```python
from build123d import *

# Parameters (mm, degrees)
F1_DEPTH = 43


with BuildPart() as f1:
    # F0 (on Front) → F1 (new body)
    with BuildSketch(Plane.XZ):
        with BuildLine():
            ThreePointArc((-7, 0), (0, -7), (7, 0))
            ThreePointArc((7, 0), (0, 7), (-7, 0))
        make_face()
        with BuildLine():
            Line((-14, 11), (-14, 0))
            Line((-14, 0), (-14, -7))
            Line((-14, -7), (-7, -14))
            Line((-7, -14), (0, -14))
            Line((0, -14), (21.066626, -14))
            ThreePointArc((21.066626, -14), (24.331862, -15.213414), (26.012265, -18.264706))
            ThreePointArc((26.012265, -18.264706), (28.349095, -26.115672), (32.788067, -33))
            Line((32.788067, -33), (38, -33))
            Line((38, -33), (67, 0))
            Line((67, 0), (67, 19))
            Line((67, 19), (65.127473, 23.242816))
            Line((65.127473, 23.242816), (41.127473, 23.242816))
            ThreePointArc((41.127473, 23.242816), (32.713444, 15.660003), (21.479572, 14.212572))
            Line((21.479572, 14.212572), (0, 18))
            Line((0, 18), (-7, 18))
            Line((-7, 18), (-14, 11))
        make_face()
        with BuildLine():
            ThreePointArc((-7, 0), (0, 7), (7, 0))
            ThreePointArc((7, 0), (0, -7), (-7, 0))
        make_face(mode=Mode.SUBTRACT)
    extrude(amount=F1_DEPTH)


solid = f1.part
```
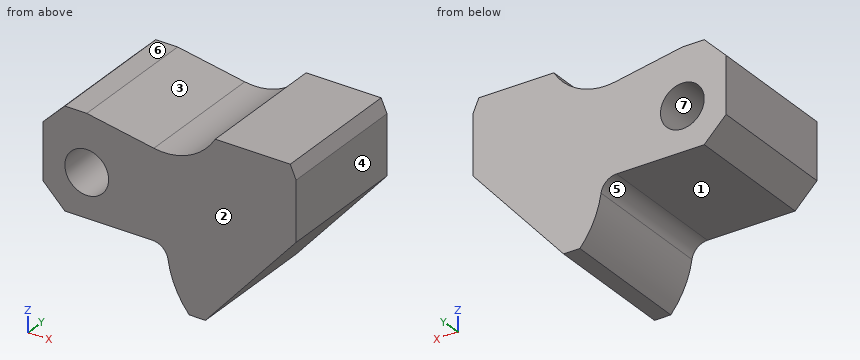
Here's how the part is built. I have some questions about the finished solid (model axes, mm). Face numbers are marked on the shaded views. A direction names the side the tool comes from. Give positions to 0.01 mm unless a question says otherwise; leave off trailing zeros. Order: outer loops, then holes, each group sorted by start corner. A loop starts at its lowest first (then second) coordinate and runs counter-clockwise, first axis right, second up. Notation, with made-up numbers: (35, 22) - (94, 22) arc R14 ccw to (94, 44) - close; hole circle Ø2 at (-8.5, -34.75). An arc over 180 degrees is marked (long way). Answer as a JSON object with one key per item and string values. Group by question number.
Item 1: If we mould it in two halves opening along Z, with no side actions, what happens to the marked faces 4, 5, 6 and 7? For each: pulls with the +Z half, pulls with the -Z half, needs draft (parallel to the pull), parting line crosses it, or undercut.
Item 2: Which directions (+Z, -Z, +X, -X, +Y, -Y) give clear straight access to the entire face, cutting with the end or side of a thin tool? Please do the marked faces 1, 2 and 3.
Item 3: If we section it at D-D on z = -27: Please give me the cut outline in (x, y).
Item 4: For P1, Ø5, axis at y = -20, z = -12.5, coming from the -X side; P2, Ø1, axis at y = -9.5, z = -25.5, coming from the -X side; P3, Ø2, axis at x = 1, y = -22.5, coming from the -Z side, each with a flat end and sliding along its axis, tell me the tip position at first contact or that it passes through.
Item 5: If we section it at B-B on z = -1: Please give me the cut outline in (x, y), and give its area (3 significant figures).
Item 6: If we section it at C-C on x = 13: Please give me the cut outline in (y, z).
Item 7: Please list where these lines run through material, in increasing order: probe 1 along Z at (x, y) = (0, -30); probe 2 along X at (y, z) = (-24, 0); probe 3 along X at (y, z) = (-32.5, 5).
Item 8: If we section it at A-A on y = -4: Please give me the cut outline in (x, z).
Result set:
{
 "1": {"face 4": "needs draft", "face 5": "pulls with the -Z half", "face 6": "pulls with the +Z half", "face 7": "undercut"},
 "2": {"face 1": "-Z, -X, +Y, -Y", "face 2": "+Z, -Z, +X, -X, -Y", "face 3": "+Z, +Y, -Y"},
 "3": {"outline": "(28.77, -43) - (43.27, -43) - (43.27, 0) - (28.77, 0) - close"},
 "4": {"P1": "x = -11", "P2": "x = 27.86", "P3": "z = -14"},
 "5": {"outline": "(-14, -43) - (-6.93, -43) - (-6.93, 0) - (-14, 0) - close; (6.93, -43) - (66.12, -43) - (66.12, 0) - (6.93, 0) - close", "area": "2,850 mm²"},
 "6": {"outline": "(-43, -14) - (0, -14) - (0, 15.71) - (-43, 15.71) - close"},
 "7": {"probe 1": "-14 to -7, 7 to 18", "probe 2": "-14 to -7, 7 to 67", "probe 3": "-14 to -4.9, 4.9 to 67"},
 "8": {"outline": "(-14, -7) - (-7, -14) - (21.07, -14) arc R5 cw to (26.01, -18.26) arc R29 ccw to (32.79, -33) - (38, -33) - (67, 0) - (67, 19) - (65.13, 23.24) - (41.13, 23.24) arc R19 cw to (21.48, 14.21) - (0, 18) - (-7, 18) - (-14, 11) - close; hole circle Ø14 at (0, 0)"}
}
